from build123d import *
from build123d.topology import SkipClean

# Parameters (mm, degrees)
SKETCH1_R           = 1.6
BOSS_EXTRUDE1_DEPTH = 2.5
BOSS_EXTRUDE2_START = -2.5
SKETCH1_3_R         = 1.6
SKETCH1_3_R_2       = 1.65
BOSS_EXTRUDE2_DEPTH = 2.5
BOSS_EXTRUDE3_START = 1
SKETCH4_R           = 2.65
SKETCH4_R_2         = 1.65
BOSS_EXTRUDE3_DEPTH = 1


with BuildPart() as part:
    # Sketch1 → Boss-Extrude1 (new body)
    with BuildSketch(Plane(origin=(0, 0, 0), x_dir=(0, 0, -1), z_dir=(1, 0, 0))):
        Polygon((0, 5.883419246), (0, 0), (15, 0), (15, 30), (0, 30), (0, 9.116580754), (2.8, 10.733161507), (5.6, 9.116580754), (5.6, 5.883419246), (2.8, 4.266838493), align=None)
        with Locations((7.5, 18)):
            Circle(SKETCH1_R, mode=Mode.SUBTRACT)
        with Locations((7.5, 25)):
            Circle(SKETCH1_R, mode=Mode.SUBTRACT)
    extrude(amount=BOSS_EXTRUDE1_DEPTH)

    # Sketch1<3> → Boss-Extrude2 (add)
    # profile 1 of 7: a face of its own
    with SkipClean():  # the faces are left unmerged after this step: merging them gives an invalid solid
        with BuildSketch(Plane(origin=(0, 0, 0), x_dir=(0, 0, -1), z_dir=(1, 0, 0)).offset(BOSS_EXTRUDE2_START)):
            Polygon((0, 5.883419246), (0, 0), (15, 0), (15, 30), (0, 30), (0, 9.116580754), (2.8, 10.733161507), (5.6, 9.116580754), (5.6, 5.883419246), (2.8, 4.266838493), align=None)
            with Locations((7.5, 7.5)):
                Circle(SKETCH1_3_R, mode=Mode.SUBTRACT)
            with BuildLine():
                ThreePointArc((6.2510004, 19), (6.970094046, 21.509701851), (9.1, 20))
                ThreePointArc((9.1, 20), (9.009701851, 19.470094046), (8.7489996, 19))
                ThreePointArc((8.7489996, 19), (9.009701851, 18.529905954), (9.1, 18))
                ThreePointArc((9.1, 18), (6.970094046, 16.490298149), (6.2510004, 19))
            make_face(mode=Mode.SUBTRACT)
            with Locations((7.5, 25)):
                Circle(SKETCH1_3_R, mode=Mode.SUBTRACT)
        # profile 2 of 7: a face of its own
        with BuildSketch(Plane(origin=(0, 0, 0), x_dir=(0, 0, -1), z_dir=(1, 0, 0)).offset(BOSS_EXTRUDE2_START)):
            Polygon((0, 5.883419246), (0, 0), (15, 0), (15, 30), (0, 30), (0, 9.116580754), (2.8, 10.733161507), (5.6, 9.116580754), (5.6, 5.883419246), (2.8, 4.266838493), align=None)
            with Locations((7.5, 7.5)):
                Circle(SKETCH1_3_R, mode=Mode.SUBTRACT)
            with BuildLine():
                ThreePointArc((6.2510004, 19), (6.970094046, 21.509701851), (9.1, 20))
                ThreePointArc((9.1, 20), (9.009701851, 19.470094046), (8.7489996, 19))
                ThreePointArc((8.7489996, 19), (9.009701851, 18.529905954), (9.1, 18))
                ThreePointArc((9.1, 18), (6.970094046, 16.490298149), (6.2510004, 19))
            make_face(mode=Mode.SUBTRACT)
            with Locations((7.5, 25)):
                Circle(SKETCH1_3_R, mode=Mode.SUBTRACT)
        # profile 3 of 7: a face of its own
        with BuildSketch(Plane(origin=(0, 0, 0), x_dir=(0, 0, -1), z_dir=(1, 0, 0)).offset(BOSS_EXTRUDE2_START)):
            Polygon((0, 9.116580754), (0, 5.883419246), (2.8, 4.266838493), (5.6, 5.883419246), (5.6, 9.116580754), (2.8, 10.733161507), align=None)
            with Locations((2.8, 7.5)):
                Circle(SKETCH1_3_R_2, mode=Mode.SUBTRACT)
        # profile 4 of 7: a face of its own
        with BuildSketch(Plane(origin=(0, 0, 0), x_dir=(0, 0, -1), z_dir=(1, 0, 0)).offset(BOSS_EXTRUDE2_START)):
            with Locations((7.5, 7.5)):
                Circle(SKETCH1_3_R)
        # profile 5 of 7: a face of its own
        with BuildSketch(Plane(origin=(0, 0, 0), x_dir=(0, 0, -1), z_dir=(1, 0, 0)).offset(BOSS_EXTRUDE2_START)):
            with Locations((7.5, 7.5)):
                Circle(SKETCH1_3_R)
        # profile 6 of 7: a face of its own
        with BuildSketch(Plane(origin=(0, 0, 0), x_dir=(0, 0, -1), z_dir=(1, 0, 0)).offset(BOSS_EXTRUDE2_START)):
            with BuildLine():
                ThreePointArc((8.7489996, 19), (9.009701851, 19.470094046), (9.1, 20))
                ThreePointArc((9.1, 20), (6.970094046, 21.509701851), (6.2510004, 19))
                ThreePointArc((6.2510004, 19), (7.5, 19.6), (8.7489996, 19))
            make_face()
        # profile 7 of 7: a face of its own
        with BuildSketch(Plane(origin=(0, 0, 0), x_dir=(0, 0, -1), z_dir=(1, 0, 0)).offset(BOSS_EXTRUDE2_START)):
            with BuildLine():
                ThreePointArc((8.7489996, 19), (9.009701851, 19.470094046), (9.1, 20))
                ThreePointArc((9.1, 20), (6.970094046, 21.509701851), (6.2510004, 19))
                ThreePointArc((6.2510004, 19), (7.5, 19.6), (8.7489996, 19))
            make_face()
        extrude(amount=BOSS_EXTRUDE2_DEPTH)

    # Sketch4 → Boss-Extrude3 (add)
    with BuildSketch(Plane.ZY.offset(2.5).offset(BOSS_EXTRUDE3_START)):
        with Locations(Location((-2.8, 7.5, 0), (0, 0, 180))):
            Circle(SKETCH4_R)
        with Locations(Location((-2.8, 7.5, 0), (0, 0, 180))):
            Circle(SKETCH4_R_2, mode=Mode.SUBTRACT)
    extrude(amount=-BOSS_EXTRUDE3_DEPTH)


solid = part.part
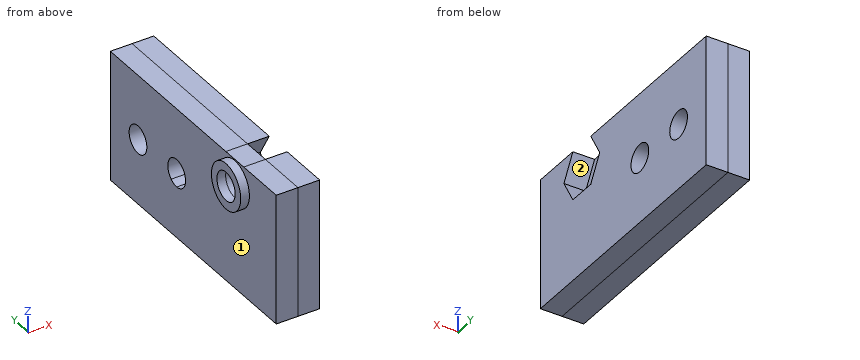
Geometry: final body of the model. Coordinates: model frame, mm. Face numbers are marked on the shaded views. Coordinates: 2 decimals unless noted, no trailing zeros. Order: outer loops, then holes, each group sorted by start corner. A loop starts at its lowest first (then second) coordinate and runs counter-clockwise, first axis right, second up. Notation, with made-up numbers: M 16.25,-6 L 38.25,-6 A17 cw 38.25,23 Z; hole C 8,43 d7. An arc over 180 degrees is marked long. One line per question, with ' | ' between items. Start each with the question number.
Item 1: Ray query, probe 1 along Y at (x, z) = (0.8, -7.5); probe 2 along Y at (x, z) = (-1.75, -2.8); probe 3 along Y at (x, z) = (-2.95, -2.8). Return the intervals inside material, ascending. Write a range as [from, to].
Item 2: Draft query along Y for the marked faces 1 and 2. Return one class per face: released by +Y, released by -Y, zero draft, split by the parting line, or undercut.
Item 3: Cut plane C-C, the plane z = -1.75. Return the cut outline in (x, y), then the cut area to 3 significant figures.
Item 4: Pin query (flat end, axial travel): pin 1 Ø7.5 at (y, z) = (16.5, -9.5) entering from -X. Return the tip coordinate at first contact, or that it passes through.
Item 5: Cut plane B-B, the plane x = -0.6. Return the cut outline in (y, z).
Item 6: Cut plane D-D, the plane y = 5.25. Return the cut outline in (x, z), then the cut area to 3 significant figures.
Item 7: Cut plane A-A, the plane y = 25. Return the cut outline in (x, z), then the cut area to 3 significant figures.
A:
1) probe 1: y = [0, 16.4], [19.6, 23.4], [26.6, 30] | probe 2: y = [0, 5.85], [9.15, 30] | probe 3: y = [4.85, 5.85], [9.15, 10.15]
2) face 1: zero draft | face 2: undercut
3) outline: M -3.5,5.07 L -2.5,5.07 L -2.5,0 L 2.5,0 L 2.5,4.87 L 0,4.87 L 0,6.23 L -3.5,6.23 Z; M -3.5,8.77 L 0,8.77 L 0,10.13 L 2.5,10.13 L 2.5,30 L -2.5,30 L -2.5,9.93 L -3.5,9.93 Z | area: 133 mm2
4) pin 1: stops at x = -2.5
5) outline: M 0,-15 L 30,-15 L 30,0 L 0,0 Z; hole C 7.5,-2.8 d3.3; hole C 18,-7.5 d3.2; hole C 25,-7.5 d3.2
6) outline: M -3.5,-4.2 L -2.5,-4.2 L -2.5,-15 L 2.5,-15 L 2.5,-4.5 L 0,-4.5 L 0,-1.1 L 2.5,-1.1 L 2.5,0 L -2.5,0 L -2.5,-1.4 L -3.5,-1.4 Z | area: 69.3 mm2
7) outline: M -2.5,-15 L 2.5,-15 L 2.5,-9.1 L -2.5,-9.1 Z; M -2.5,-5.9 L 2.5,-5.9 L 2.5,0 L -2.5,0 Z | area: 59.0 mm2
